Autodesk Inventor part; units mm, degrees
ref_plane "YZ Plane" through (0, 0, 0) normal (1, 0, 0) x (0, 1, 0)
ref_plane "XZ Plane" through (0, 0, 0) normal (0, 1, 0) x (-1, 0, 0)
ref_plane "XY Plane" through (0, 0, 0) normal (0, 0, 1) x (1, 0, 0)
sketch "Sketch1" plane through (0, 0, 0) normal (0, 0, 1) x (1, 0, 0)
  line L0 (3.85, 3.85) -> (-3.85, 3.85)
  line L1 (-3.85, 3.85) -> (-3.85, -5.5)
  line L2 (-3.85, -5.5) -> (3.85, -5.5)
  line L3 (3.85, -5.5) -> (3.85, 3.85)
  point P0 (0, 0)
  dimension "d0" = 7.7
  dimension "d1" = 3.85
  dimension "d2" = 3.85
  dimension "d3" = 5.5
extrude "Extrusion1" add sketch "Sketch1" against normal blind 10
sketch "Sketch2" plane through (0, 0, 0) normal (0, 0, 1) x (1, 0, 0)
  circle A0 centre (0, 0) radius 3
  dimension "d6" = 6
extrude "Extrusion2" add sketch "Sketch2" along normal blind 5
sketch "Sketch3" plane through (0, 0, 5) normal (0, 0, 1) x (1, 0, 0)
  circle A0 centre (0, 0) radius 3
  circle A1 centre (0, 0) radius 2.5
  dimension "d9" = 5
extrude "Extrusion3" add sketch "Sketch3" along normal blind 6.5 contours A1
sketch "Sketch4" plane through (0, 0, 0) normal (1, 0, 0) x (0, 1, 0)
  line L0 (1, 13.5) -> (-1, 13.5)
  line L1 (-1, 13.5) -> (-1, 7.5)
  line L2 (-1, 7.5) -> (1, 7.5)
  line L3 (1, 7.5) -> (1, 13.5)
  line L4 (2.5, 11.5) -> (-2.5, 11.5)
  line L5 (0, 11.5) -> (1, 13.5) construction
  line L6 (0, 11.5) -> (-1, 13.5) construction
  point P0 (0, 0)
  dimension "d12" = 2
  dimension "d13" = 4
  dimension "d14" = 2
extrude "Extrusion4" cut sketch "Sketch4" along normal through all both and the other way through all
sketch "Sketch5" plane through (0, 0, 0) normal (0, 0, 1) x (1, 0, 0)
  circle A0 centre (0, 0) radius 3
  circle A1 centre (0, 0) radius 1.75
  dimension "d17" = 3.5
extrude "Extrusion5" add sketch "Sketch5" along normal blind 21 contours A1
sketch "Sketch6" plane through (0, 0, 21) normal (0, 0, 1) x (1, 0, 0)
  circle A0 centre (0, 0) radius 1.75
  line L0 (-2, -2.75) -> (2, -2.75)
  line L1 (2, -2.75) -> (2, -0.75)
  line L2 (2, -0.75) -> (-2, -0.75)
  line L3 (-2, -0.75) -> (-2, -2.75)
  dimension "d21" = 2.5
  dimension "d22" = 2
  dimension "d23" = 2
  dimension "d24" = 2
extrude "Extrusion6" cut sketch "Sketch6" against normal blind 6 contours L2 A0 | A0 L2 L1 L0 L3 picked at (0.0313, -1.2733)
chamfer "Chamfer1" distance 0.5 angle 45 5 edges at (1.7073, -0.3844, 21) (-0.3844, 1.7073, 21) (0, 2.5, 11.5) (0, -2.5, 11.5) (-3, 0, 5)
sketch "Sketch7" plane through (-3.85, -5.5, 0) normal (0, -1, 0) x (1, 0, 0)
  line L0 (0, 0) -> (7.7, 0)
  line L1 (0, 0) -> (0, -10)
  line L2 (7.7, -10) -> (0, -10)
  line L3 (7.7, 0) -> (7.7, -10)
  circle A0 centre (3.85, -3.8) radius 0.4
  circle A1 centre (3.85, -8.3) radius 0.4
  circle A2 centre (5.85, -3.8) radius 0.4
  circle A3 centre (5.85, -8.3) radius 0.4
  circle A4 centre (1.85, -8.3) radius 0.4
  circle A5 centre (1.85, -3.8) radius 0.4
  line L4 (3.85, -3.8) -> (1.85, -3.8) construction
  line L5 (1.85, -8.3) -> (1.85, -3.8) construction
  line L6 (1.85, -8.3) -> (3.85, -8.3) construction
  line L7 (3.85, -8.3) -> (5.85, -8.3) construction
  line L8 (5.85, -8.3) -> (5.85, -3.8) construction
  line L9 (5.85, -3.8) -> (3.85, -3.8) construction
  point P0 (3.85, 0)
  dimension "d30" = 0.8
  dimension "d31" = 3.8
  dimension "d32" = 4.5
  dimension "d33" = 2
  dimension "d34" = 2
  dimension "d37" = 3.85
  dimension "d38" = 1.7
extrude "Extrusion7" add sketch "Sketch7" along normal blind 3 contours A0 | A1 | A2 | A3 | A4 | A5
thread "Thread1"
properties part number "P082D"
Part model, mm, in its own coordinate system. A direction names the side the tool comes from. Round coordinates to 2 decimals unless told otherwise and drop trailing zeros. Loops run counter-clockwise (first coordinate to the right, second up) from the corner with the lowest first, then second, coordinate; pieces in that order, holes last.
1. Flat gauge pins, fed straight in: pin 1 (0.7 mm diameter, centred on x = 1.5, z = 10, fed in from -Y); pin 2 (2 mm diameter, centred on x = -1.5, y = -6, fed in from +Z); pin 3 (1.1 mm diameter, centred on x = 0, y = -1.5, fed in from +Z). Where does each tip first touch, or does it go through?
Solutions:
pin 1: stops at y = -2.22
pin 2: stops at z = 0
pin 3: stops at z = 15
2. 3-axis set-ups, long thin cutter, end or side, ignore diameter. For faces 1 (the face through (-0.09, -6.98, -3.41)), 2 (the face through (0, -1, 15)), 3 (the face through (-3.85, -1, -5)): which of +Z, -Z, +X, -X, +Y, -Y reach the whole face in a straight line?
Solutions:
face 1: -Y
face 2: +Z, +X, -X, -Y
face 3: +Z, -Z, -X, +Y, -Y
3. Two-plate mould, pull along Y, no slides. Class faces 4 (the face through (-0.04, 1.39, 20.86)), 5 (the face through (-2, 0, 7.5)), 6 (the face through (-0.03, 2.14, 11.36)): pulls with the +Y half, pulls with the -Y half, needs draft (parallel to the pull), parting line crosses it, or undercut.
Solutions:
face 4: parting line crosses it
face 5: undercut
face 6: pulls with the +Y half
4. Slice it at C-C (z = -3.8). Give the cut face in (x, y), and give its area (3 significant figures).
Solutions:
outline: (-3.85, -5.5) - (-2.4, -5.5) - (-2.4, -8.5) - (-1.6, -8.5) - (-1.6, -5.5) - (-0.4, -5.5) - (-0.4, -8.5) - (0.4, -8.5) - (0.4, -5.5) - (1.6, -5.5) - (1.6, -8.5) - (2.4, -8.5) - (2.4, -5.5) - (3.85, -5.5) - (3.85, 3.85) - (-3.85, 3.85) - close
area: 79.2 mm2
5. Slice it at A-A (y = -7). Give the cut face in (x, z).
Solutions:
outline: circle Ø0.8 at (-2, -8.3); circle Ø0.8 at (-2, -3.8); circle Ø0.8 at (0, -8.3); circle Ø0.8 at (0, -3.8); circle Ø0.8 at (2, -8.3); circle Ø0.8 at (2, -3.8)
6. Drill centre lines: line 1 along Z through (x, y) = (-3, -1.5); line 2 along Y through (x, z) = (1.5, -5.5); line 3 along Z through (x, y) = (2, -7.75). Where is each one in solid material? Low to high.
Solutions:
line 1: z = -10 to 0
line 2: y = -5.5 to 3.85
line 3: z = -8.7 to -7.9, -4.2 to -3.4
